Here's how the part is built. I have some questions about the finished solid (model axes, mm). A direction names the side the tool comes from. Round coordinates to 2 decimals unless told otherwise and drop trailing zeros. Loops run counter-clockwise (first coordinate to the right, second up) from the corner with the lowest first, then second, coordinate; pieces in that order, holes last. Notation, with made-up numbers: M 1,29.5 L 24,29.5 A25 ccw 24,57.5 Z; hole C 85.5,-13 d11. An arc over 180 degrees is marked long. Use a Markdown table: item, result.
```python
from build123d import *

# Parameters (mm, degrees)
SKETCH1_W               = 25.4
SKETCH1_H               = 50.8
SKETCH1_W_2             = 19.05
SKETCH1_H_2             = 44.45
BOSS_EXTRUDE1_DEPTH     = 304.8
SKETCH2_R               = 12.7
CUT_EXTRUDE1_DEPTH      = 1
CUT_EXTRUDE1_DEPTH_BACK = 26.4
SKETCH3_W               = 50.8
SKETCH3_H               = 55.112369071
CUT_EXTRUDE2_DEPTH      = 159.004


with BuildPart() as part:
    # Sketch1 → Boss-Extrude1 (new body)
    with BuildSketch(Plane(origin=(0, 0, 0), x_dir=(0, 0, -1), z_dir=(1, 0, 0))):
        with Locations((12.7, 25.4)):
            Rectangle(SKETCH1_W, SKETCH1_H)
        with Locations((12.7, 25.4)):
            Rectangle(SKETCH1_W_2, SKETCH1_H_2, mode=Mode.SUBTRACT)
    extrude(amount=BOSS_EXTRUDE1_DEPTH)

    # Sketch2 → Cut-Extrude1 (cut, two sides)
    with BuildSketch(Plane(origin=(0, 0, -25.4), x_dir=(-1, 0, 0), z_dir=(0, 0, -1))) as cut_extrude1_sk:
        with Locations((-279.4, 27.283270028)):
            Circle(SKETCH2_R)
    extrude(amount=CUT_EXTRUDE1_DEPTH, mode=Mode.SUBTRACT)
    extrude(cut_extrude1_sk.sketch, amount=-CUT_EXTRUDE1_DEPTH_BACK, mode=Mode.SUBTRACT)

    # Sketch3 → Cut-Extrude2 (cut)
    with BuildSketch(Plane(origin=(0, 0, -25.4), x_dir=(-1, 0, 0), z_dir=(0, 0, -1))):
        with Locations((-25.4, 23.243815465)):
            Rectangle(SKETCH3_W, SKETCH3_H)
    extrude(amount=-CUT_EXTRUDE2_DEPTH, mode=Mode.SUBTRACT)


solid = part.part
```
Q1. We'd pull the mould along Z, two halves only. Please class faces 3 (the flat face through (304.8, 24, -2)), 4 (the flat face through (176, 25, -22.225)), 5 (the flat face through (176, 3.175, -13)), 6 (the flat face through (176, 25, 0)): pulls with the +Z half, pulls with the -Z half, needs draft (parallel to the pull), parting line crosses it, or undercut.
Return value:
| item | result |
|---|---|
| face 3 | needs draft |
| face 4 | undercut |
| face 5 | undercut |
| face 6 | pulls with the +Z half |
Q2. Imagine slicing it at B-B, the plane z = -18.5. Please give me the cut outline in (x, y) (3 decimals), then the cut area to 3 significant figures.
Return value:
| item | result |
|---|---|
| outline | M 50.8,0 L 304.8,0 L 304.8,3.175 L 50.8,3.175 Z; M 50.8,47.625 L 304.8,47.625 L 304.8,50.8 L 50.8,50.8 Z |
| area | 1,610 mm^2 |
Q3. Imagine slicing it at D-D, the plane x = 195. Please give me the cut outline in (y, z) (3 decimals).
Return value:
| item | result |
|---|---|
| outline | M 0,-25.4 L 50.8,-25.4 L 50.8,0 L 0,0 Z; hole M 3.175,-22.225 L 47.625,-22.225 L 47.625,-3.175 L 3.175,-3.175 Z |
Q4. Imagine slicing it at C-C, the plane y = 45.5. Please give me the cut outline in (x, z) (3 decimals), then the cut area to 3 significant figures.
Return value:
| item | result |
|---|---|
| outline | M 50.8,-25.4 L 304.8,-25.4 L 304.8,-22.225 L 50.8,-22.225 Z; M 50.8,-3.175 L 304.8,-3.175 L 304.8,0 L 50.8,0 Z |
| area | 1,610 mm^2 |
Q5. I need wall thicknesses on line 1 (Y direction, x = 207, z = -20.75) (3 decimals); line 2 (Z direction, x = 144, y = 18) (3 decimals); line 3 (Y direction, x = 279.4, z = -2.4). Which ranges of each line are inside material? Lowest first, please. Write a range as from..to.
Return value:
| item | result |
|---|---|
| line 1 | y = 0..3.175, 47.625..50.8 |
| line 2 | z = -25.4..-22.225, -3.175..0 |
| line 3 | y = 0..14.58, 39.98..50.8 |
Q6. Imagine slicing it at A-A, the plane x = 279.4. Please give me the cut outline in (y, z) (3 decimals), then the cut area to 3 significant figures.
Return value:
| item | result |
|---|---|
| outline | M 0,-25.4 L 14.583,-25.4 L 14.583,-22.225 L 3.175,-22.225 L 3.175,-3.175 L 14.583,-3.175 L 14.583,0 L 0,0 Z; M 39.983,-25.4 L 50.8,-25.4 L 50.8,0 L 39.983,0 L 39.983,-3.175 L 47.625,-3.175 L 47.625,-22.225 L 39.983,-22.225 Z |
| area | 282 mm^2 |
Q7. For faces 1 (the flat face through (176, 25, -3.175)), 2 (the cylindrical face through (292.088, 27.842, -23.835)), which set-ups out of +Z, -Z, +X, -X, +Y, -Y let a thin tool reach every point of the face, with its end or its side?
Return value:
| item | result |
|---|---|
| face 1 | +X, -X |
| face 2 | +Z, -Z |
